from build123d import *

# Parameters (mm, degrees)
SKETCH1_W           = 7
SKETCH1_H           = 33
BOSS_EXTRUDE1_DEPTH = 13
FILLET4_R           = 0.5
SKETCH3_R           = 1.25
CUT_EXTRUDE1_DEPTH  = 22.295539439
SKETCH5_R           = 1.25
SKETCH5_W           = 12.1
SKETCH5_H           = 10.1
CUT_EXTRUDE2_DEPTH  = 23.141589825
FILLET5_R           = 0.5


with BuildPart() as part:
    # Sketch1 → Boss-Extrude1 (new body)
    with BuildSketch(Plane(origin=(0, 0, 0), x_dir=(1, 0, 0), z_dir=(0, 1, 0))):
        Rectangle(SKETCH1_W, SKETCH1_H)
    extrude(amount=BOSS_EXTRUDE1_DEPTH)

    # Fillet4
    fillet4_edges = [part.edges().sort_by_distance(p)[0] for p in [
        (0, 13, 16.5),
        (-3.5, 13, 0),
        (0, 13, -16.5),
        (3.5, 13, 0),
    ]]
    fillet(fillet4_edges, radius=FILLET4_R)

    # Sketch3 → Cut-Extrude1 (cut, through all)
    with BuildSketch(Plane(origin=(0, 13, 0), x_dir=(1, 0, 0), z_dir=(0, 1, 0))):
        with Locations(Location((1, 9.5, 0), (0, 0, 270))):
            Circle(SKETCH3_R)
        with Locations(Location((1, -9.5, 0), (0, 0, 270))):
            Circle(SKETCH3_R)
    extrude(amount=-CUT_EXTRUDE1_DEPTH, mode=Mode.SUBTRACT)

    # Sketch5 → Cut-Extrude2 (cut, through all)
    with BuildSketch(Plane.ZY.offset(3.5)):
        with Locations((-13.25, 5)):
            Circle(SKETCH5_R)
        with Locations(Location((13.25, 5, 0), (0, 0, 180))):
            Circle(SKETCH5_R)
        with Locations((0.05, 5.05)):
            Rectangle(SKETCH5_W, SKETCH5_H)
    extrude(amount=-CUT_EXTRUDE2_DEPTH, mode=Mode.SUBTRACT)

    # Fillet5
    fillet5_edges = [part.edges().sort_by_distance(p)[0] for p in [
        (0, 10.1, -6),
        (0, 10.1, 6.1),
    ]]
    fillet(fillet5_edges, radius=FILLET5_R)


solid = part.part
Geometry: final body of the model. Coordinates: model frame, mm. A direction names the side the tool comes from. Coordinates: 2 decimals unless noted, no trailing zeros. Order: outer loops, then holes, each group sorted by start corner. A loop starts at its lowest first (then second) coordinate and runs counter-clockwise, first axis right, second up.
(1) Material intervals for probe 1 along Z at (x, y) = (-2.5, 8.25); probe 2 along Z at (x, y) = (2, 12); probe 3 along X at (y, z) = (4, -9.5), sorted ascending.
(2) Section query C-C (z = -14). Return the cut outline in (x, y).
(3) Draft query along Z for faces 3 (the face through (0, 10.1, 0)), 4 (the face through (0, 4, -14)), 5 (the face through (0, 6, -16.5)), 6 (the face through (0, 0, -11)). Return one class per face: pulls with the +Z half, pulls with the -Z half, needs draft (parallel to the pull), parting line crosses it, or undercut.
(4) Section query A-A (x = 0.25). Return the cut outline in (y, z), plus the area to 3 significant figures.
(5) First-contact query: pin 1 (2 mm diameter, centred on y = 5, z = 13.25, fed in from -X). Flat tip, straight axial feed; report the tip coordinate or a pass-through.
(6) Access query for faces 1 (the face through (-3.5, 10.3, 0.2)), 2 (the face through (0, 5, -6)). Directions: +Z, -Z, +X, -X, +Y, -Y. A direction counts if a zero-diameter tool reaches every point of the face in a straight line with its end or side. Return the directions, or none.
(7) Section query D-D (x = -2.5). Return the cut outline in (y, z).
(8) Section query B-B (y = 2.75). Return the cut outline in (x, z).
Solution:
1. probe 1: z = -16.5 to -6, 6.1 to 16.5
1. probe 2: z = -16.5 to -10.25, -8.75 to 8.75, 10.25 to 16.5
1. probe 3: x = -3.5 to -0.25, 2.25 to 3.5
2. outline: (-3.5, 0) - (3.5, 0) - (3.5, 4) - (-3.5, 4) - close; (-3.5, 6) - (3.5, 6) - (3.5, 12.5) arc R0.5 ccw to (3, 13) - (-3, 13) arc R0.5 ccw to (-3.5, 12.5) - close
3. face 3: undercut
3. face 4: undercut
3. face 5: pulls with the -Z half
3. face 6: needs draft
4. outline: (0, -16.5) - (12.5, -16.5) arc R0.5 ccw to (13, -16) - (13, -10.5) - (0, -10.5) - close; (0, -8.5) - (13, -8.5) - (13, 8.5) - (0, 8.5) - (0, 6.1) - (9.6, 6.1) arc R0.5 cw to (10.1, 5.6) - (10.1, -5.5) arc R0.5 cw to (9.6, -6) - (0, -6) - close; (0, 10.5) - (13, 10.5) - (13, 16) arc R0.5 ccw to (12.5, 16.5) - (0, 16.5) - close; hole circle Ø2.5 at (5, -13.25); hole circle Ø2.5 at (5, 13.25)
4. area: 245 mm2
5. pin 1: passes through
6. face 1: +Z, -Z, -X, +Y, -Y
6. face 2: +X, -X, -Y
7. outline: (0, -16.5) - (12.5, -16.5) arc R0.5 ccw to (13, -16) - (13, 16) arc R0.5 ccw to (12.5, 16.5) - (0, 16.5) - (0, 6.1) - (9.6, 6.1) arc R0.5 cw to (10.1, 5.6) - (10.1, -5.5) arc R0.5 cw to (9.6, -6) - (0, -6) - close; hole circle Ø2.5 at (5, -13.25); hole circle Ø2.5 at (5, 13.25)
8. outline: (-3.5, -16.5) - (3.5, -16.5) - (3.5, -6) - (-3.5, -6) - close; (-3.5, 6.1) - (3.5, 6.1) - (3.5, 16.5) - (-3.5, 16.5) - close; hole circle Ø2.5 at (1, -9.5); hole circle Ø2.5 at (1, 9.5)
